Design review of the part built by this model. Coordinates are the model's own, in mm. Round coordinates to 2 decimals unless told otherwise and drop trailing zeros. Loops run counter-clockwise (first coordinate to the right, second up) from the corner with the lowest first, then second, coordinate; pieces in that order, holes last. Notation, with made-up numbers: M 0,24.5 L 24,24.5 A24 cw 24,41.5 Z; hole C 77.5,52.5 d11. An arc over 180 degrees is marked long. One line per item, written item: value. Start each with the question number.
Item 1: We need section A-A (z = 1). Write out the cut boundary in (x, y).
Item 2: We need section C-C (y = 2.25). Write out the cut boundary in (x, z).
Item 3: We need section B-B (y = 0). Write out the cut boundary in (x, z), then the cut area to 3 significant figures.
Item 4: We need section D-D (z = 6.5). Write out the cut boundary in (x, y), then the cut area to 3 significant figures.
Item 5: For line 1 along Y through (x, z) = (-3.25, 2.25); line 2 along Y through (x, z) = (0.75, 1.25); line 3 along X through (y, z) = (-1.75, 5.5), list the stretches that pass through material, from the lowest coordinate up.
Item 6: Clearance check with a flat-ended pin moving along its axis: pin 1 (2 mm diameter, centred on y = 4, z = 2, fed in from -X). State where the tip first meets the part, or that it passes through.
Item 7: Mouldability with a two-part tool opening along Y and no side actions: class faces 1 (the cylindrical face through (-3.868, -2.966, 3.451)), 2 (the flat face through (3.35, -5.913, 2.712)), 3 (the flat face through (3.446, 5.858, 2.712)), 4 (the cylindrical face through (6.368, 0.055, 6.549)) as released by +Y, released by -Y, zero draft, split by the parting line, or undercut.
from build123d import *

# Parameters (mm, degrees)
F0_R     = 4.874108
F1_DEPTH = 7
F2_R     = 1.5


with BuildPart() as f1:
    # F0 (on Top) → F1 (new body)
    with BuildSketch(Plane.XY):
        Polygon((6.795984, 3.923663), (0, 7.847326), (-6.795984, 3.923663), (-6.795984, -3.923663), (0, -7.847326), (6.795984, -3.923663), align=None)
        Circle(F0_R, mode=Mode.SUBTRACT)
    extrude(amount=F1_DEPTH)

    # F2
    f2_edges = [f1.edges().sort_by_distance(p)[0] for p in [
        (6.795984, 0, 7),
        (3.397992, -5.885494, 7),
        (-3.397992, -5.885494, 7),
        (3.397992, 5.885494, 7),
        (-6.795984, 0, 7),
        (-3.397992, 5.885494, 7),
    ]]
    fillet(f2_edges, radius=F2_R)


solid = f1.part
A:
1. outline: M -6.8,-3.92 L 0,-7.85 L 6.8,-3.92 L 6.8,3.92 L 0,7.85 L -6.8,3.92 Z; hole C 0,0 d9.75
2. outline: M -6.8,0 L -4.32,0 L -4.32,7 L -5.3,7 A1.5 ccw -6.8,5.5 Z; M 4.32,0 L 6.8,0 L 6.8,5.5 A1.5 ccw 5.3,7 L 4.32,7 Z
3. outline: M -6.8,0 L -4.87,0 L -4.87,7 L -5.3,7 A1.5 ccw -6.8,5.5 Z; M 4.87,0 L 6.8,0 L 6.8,5.5 A1.5 ccw 5.3,7 L 4.87,7 Z
3. area: 25.9 mm2
4. outline: M -6.41,-3.7 L 0,-7.41 L 6.41,-3.7 L 6.41,3.7 L 0,7.41 L -6.41,3.7 Z; hole C 0,0 d9.75
4. area: 67.9 mm2
5. line 1: -5.97 to -3.63, 3.63 to 5.97
5. line 2: -7.41 to -4.82, 4.82 to 7.41
5. line 3: -6.8 to -4.55, 4.55 to 6.8
6. pin 1: x = -6.8
7. face 1: undercut
7. face 2: released by -Y
7. face 3: released by +Y
7. face 4: zero draft
